Geometry check sheet. Reference: the model listing, model coordinates, mm. A direction names the side the tool comes from. Give positions to 0.01 mm unless a question says otherwise; leave off trailing zeros. Write each loop counter-clockwise with the first axis right and the second up, starting at its lowest first coordinate (ties: lowest second). Pieces come first, ordered by that corner, then holes. Notation, with made-up numbers: (18.5, 71.5) -> (37.5, 71.5) arc R10 cw to (37.5, 88.5) -> close; hole circle Ø10 at (-30.5, 36.5). An arc over 180 degrees is marked (long way). Write item = value, one per line. Start each with the question number.
1. Cross-section at B-B, the plane z = -31.75. Record the cut outline in (x, y) (1 decimal).
2. Thickness scan on line 1 along Y through (x, z) = (20.25, -15); line 2 along X through (y, z) = (21.75, -11); line 3 along Y through (x, z) = (29.5, -17). Record the ranges inside material, lowest first.
3. Depth check by flat-ended pin: P1, Ø2, axis at x = -18.5, y = 13.5, coming from the -Z side; P2, Ø5.5, axis at x = 30.16, z = 31.75, coming from the +Y side; P3, Ø4.5, axis at y = 15.5, z = 0.5, coming from the -X side. Enter the tip coordinate at first touch or a pass-through.
4. Set-up check for faces 1 (the flat face through (24.519, 18, 0)), 2 (the flat face through (-19, 16, 24.1)), 3 (the cylindrical face through (14.52, 16.1, 23.05)), 4 (the flat face through (-19, 16, -24.1)): record each of +Z, -Z, +X, -X, +Y, -Y from which the full face is reachable in a straight line by a thin tool's end or side.
5. Cross-section at C-C, the plane y = 23.75. Record the cut outline in (x, z) (3 decimals).
6. Cross-section at A-A, the plane y = 17.4. State how many separate pieces and enclosed holes the cut face has, plus the area to 3 significant figures.
7. Cross-section at D-D, the plane z = -1.5. Record the cut outline in (x, y) (3 decimals), plus the area to 3 significant figures.
8. Mould release check, pull along X, two halves, no side actions. Record for faces 5 (the cylindrical face through (-31.829, 5.07, 33.028)), 6 (the flat face through (34.925, 5, 0)), 7 (the cylindrical face through (-23.52, 15.88, -23.05)): pulls with the +X half, pulls with the -X half, needs draft (parallel to the pull), parting line crosses it, or undercut.
```python
from build123d import *

# Parameters (mm, degrees)
BOSS_EXTRUDE1_DEPTH         = 38.1
SKETCH2_W                   = 49.038
SKETCH2_H                   = 14
CUT_EXTRUDE1_DEPTH          = 15.4
FILLET1_R                   = 3.5
TAP_DRILL_FOR_M5X0_8_TAP2_D = 4.2
TAP_DRILL_FOR_M5X0_8_TAP3_D = 4.2
CHAMFER1_SIZE               = 3.175
FILLET4_R                   = 5


with BuildPart() as part:
    # Sketch1 → Boss-Extrude1 (new, symmetric)
    with BuildSketch(Plane.XY):
        Polygon((-24.519, 25.4), (-24.519, 10), (-34.925, 10), (-34.925, 0), (34.925, 0), (34.925, 10), (24.519, 10), (24.519, 25.4), (13.519, 25.4), (13.519, 10), (-13.519, 10), (-13.519, 25.4), align=None)
    extrude(amount=BOSS_EXTRUDE1_DEPTH, both=True)

    # Sketch2 → Cut-Extrude1 (cut)
    with BuildSketch(Plane(origin=(0, 25.4, 0), x_dir=(1, 0, 0), z_dir=(0, 1, 0))):
        with Locations((0, 31.1)):
            Rectangle(SKETCH2_W, SKETCH2_H)
        with Locations((0, -31.1)):
            Rectangle(SKETCH2_W, SKETCH2_H)
    extrude(amount=-CUT_EXTRUDE1_DEPTH, mode=Mode.SUBTRACT)

    # Fillet1
    fillet1_edges = [part.edges().sort_by_distance(p)[0] for p in [
        (-13.519, 17.7, -24.1),
        (13.519, 17.7, -24.1),
        (24.519, 17.7, -24.1),
        (-24.519, 17.7, -24.1),
        (-13.519, 17.7, 24.1),
        (13.519, 17.7, 24.1),
        (-24.519, 17.7, 24.1),
        (24.519, 17.7, 24.1),
    ]]
    fillet(fillet1_edges, radius=FILLET1_R)

    # Tap Drill for M5x0.8 Tap2 (through all)
    with Locations(Plane(origin=(0, 0, 0), x_dir=(-1, 0, 0), z_dir=(0, -1, 0))):
        with Locations((-30.1625, 31.75), (30.1625, 31.75), (30.1625, -31.75), (-30.1625, -31.75)):
            Hole(TAP_DRILL_FOR_M5X0_8_TAP2_D / 2)

    # Tap Drill for M5x0.8 Tap3 (through all)
    with Locations(Plane.ZY.offset(24.519)):
        with Locations((-15, 17.4), (15, 17.4)):
            Hole(TAP_DRILL_FOR_M5X0_8_TAP3_D / 2)

    # Chamfer1
    # the kernel refuses this chamfer: 3.175 mm, written as the material it takes off along each edge
    with BuildSketch(Plane(origin=(29.184093487, 25.4, -24.1), x_dir=(0, -0.9996219169112968, -0.027495876610586726), z_dir=(-1, 0, 0)), Plane(origin=(-8.853906513, 25.4, 24.1), x_dir=(0, 0.027495876610586726, -0.9996219169112968), z_dir=(-1, 0, 0))) as chamfer1_piece_1:
        Polygon((CHAMFER1_SIZE * 0.999621916911, CHAMFER1_SIZE * 0.0274958766106), (-CHAMFER1_SIZE * 0.0274958766106, CHAMFER1_SIZE * 0.999621916911), (0, 0), align=None)
    extrude(amount=20.330186974, mode=Mode.SUBTRACT)
    with BuildSketch(Plane(origin=(29.184093487, 25.4, 24.1), x_dir=(0, -0.9996219169112968, 0.027495876610586726), z_dir=(-1, 0, 0)), Plane(origin=(-8.853906513, 25.4, -24.1), x_dir=(0, 0.027495876610586726, 0.9996219169112968), z_dir=(-1, 0, 0))) as chamfer1_piece_2:
        Polygon((CHAMFER1_SIZE * 0.999621916911, -CHAMFER1_SIZE * 0.0274958766106), (-CHAMFER1_SIZE * 0.0274958766106, -CHAMFER1_SIZE * 0.999621916911), (0, 0), align=None)
    extrude(amount=20.330186974, mode=Mode.SUBTRACT)

    # Fillet4
    fillet4_edges = [part.edges().sort_by_distance(p)[0] for p in [
        (-34.925, 5, 38.1),
        (34.925, 5, -38.1),
        (-34.925, 5, -38.1),
        (34.925, 5, 38.1),
    ]]
    fillet(fillet4_edges, radius=FILLET4_R)


solid = part.part
```
Answers:
q1.outline = (-34.9, 0) -> (-32.3, 0) -> (-32.3, 10) -> (-34.9, 10) -> close; (-28.1, 0) -> (28.1, 0) -> (28.1, 10) -> (-28.1, 10) -> close; (32.3, 0) -> (34.9, 0) -> (34.9, 10) -> (32.3, 10) -> close
q2.line_1 = 0 to 15.3, 19.5 to 25.4
q2.line_2 = -24.52 to -13.52, 13.52 to 24.52
q2.line_3 = 0 to 10
q3.P1 = -24.1
q3.P2 = 10
q3.P3 = -24.52
q4.face_1 = +Z, -Z, +X, +Y
q4.face_2 = +Z, +X, -X, +Y
q4.face_3 = +Z, +Y
q4.face_4 = -Z, +X, -X, +Y
q5.outline = (-24.519, -20.6) arc R3.5 ccw to (-23.909, -22.575) -> (-14.129, -22.575) arc R3.5 ccw to (-13.519, -20.6) -> (-13.519, 20.6) arc R3.5 ccw to (-14.129, 22.575) -> (-23.909, 22.575) arc R3.5 ccw to (-24.519, 20.6) -> close; (13.519, -20.6) arc R3.5 ccw to (14.129, -22.575) -> (23.909, -22.575) arc R3.5 ccw to (24.519, -20.6) -> (24.519, 20.6) arc R3.5 ccw to (23.909, 22.575) -> (14.129, 22.575) arc R3.5 ccw to (13.519, 20.6) -> close
q6.separate_pieces = 6
q6.enclosed_holes = 0
q6.area = 855 mm^2
q7.outline = (-34.925, 0) -> (34.925, 0) -> (34.925, 10) -> (24.519, 10) -> (24.519, 25.4) -> (13.519, 25.4) -> (13.519, 10) -> (-13.519, 10) -> (-13.519, 25.4) -> (-24.519, 25.4) -> (-24.519, 10) -> (-34.925, 10) -> close
q7.area = 1,040 mm^2
q8.face_5 = undercut
q8.face_6 = pulls with the +X half
q8.face_7 = pulls with the -X half
